Autodesk Inventor part; units mm, degrees
ref_plane "YZ Plane" through (0, 0, 0) normal (1, 0, 0) x (0, 1, 0)
ref_plane "XZ Plane" through (0, 0, 0) normal (0, 1, 0) x (-1, 0, 0)
ref_plane "XY Plane" through (0, 0, 0) normal (0, 0, 1) x (1, 0, 0)
sketch "Sketch1" plane through (0, 0, 0) normal (0, 1, 0) x (-1, 0, 0)
  line L0 (141, -70.5) -> (-141, -70.5)
  line L1 (-141, -70.5) -> (-141, 70.5)
  line L2 (-141, 70.5) -> (141, 70.5)
  line L3 (141, 70.5) -> (141, -70.5)
  line L4 (141, -70.5) -> (-141, 70.5) construction
  line L5 (-141, -70.5) -> (141, 70.5) construction
  point P0 (0, 0)
  dimension "d0" = 282
  dimension "d1" = 141
extrude "RectangleFace" add sketch "Sketch1" along normal blind 15
sketch "Sketch2" plane through (0, 15, 0) normal (0, 1, 0) x (1, 0, 0)
  line L0 (141, 70.5) -> (-141, 70.5)
  line L1 (0, 70.5) -> (0, -11.1)
  line L2 (0, -11.1) -> (-82, -11.1)
  line L3 (-122, 11.4) -> (-42, 11.4)
  line L4 (-42, 11.4) -> (-42, -33.6)
  line L5 (-42, -33.6) -> (-122, -33.6)
  line L6 (-122, -33.6) -> (-122, 11.4)
  line L7 (-122, 11.4) -> (-42, -33.6) construction
  line L8 (-42, 11.4) -> (-122, -33.6) construction
  point P0 (0, 0)
  dimension "d4" = 81.6
  dimension "d5" = 82
  dimension "d6" = 80
  dimension "d7" = 45
extrude "RectangularCut" cut sketch "Sketch2" against normal blind 15
sketch "Sketch3" plane through (0, 15, 0) normal (0, 1, 0) x (1, 0, 0)
  line L0 (-42, 11.4) -> (-122, 11.4)
  line L1 (-82, 11.4) -> (-82, 29.4)
  line L2 (-122, -33.6) -> (-42, -33.6)
  line L3 (-82, -33.6) -> (-82, -46.1)
  line L4 (-82, 29.4) -> (-74, 29.4)
  line L5 (-82, 29.4) -> (-90, 29.4)
  line L6 (-82, -46.1) -> (-74, -46.1)
  line L7 (-82, -46.1) -> (-90, -46.1)
  circle A0 centre (-74, -46.1) radius 1.75
  circle A1 centre (-90, -46.1) radius 1.75
  circle A2 centre (-74, 29.4) radius 1.75
  circle A3 centre (-90, 29.4) radius 1.75
  point P0 (0, 0)
  dimension "d10" = 18
  dimension "d11" = 12.5
  dimension "d12" = 8
  dimension "d13" = 8
  dimension "d14" = 8
  dimension "d15" = 8
  dimension "d16" = 3.5
  dimension "d17" = 3.5
  dimension "d18" = 3.5
  dimension "d19" = 3.5
extrude "AxleSupportHoles" cut sketch "Sketch3" against normal blind 15
sketch "Sketch4" plane through (0, 15, 0) normal (0, 1, 0) x (1, 0, 0)
  line L0 (141, 70.5) -> (-141, 70.5)
  line L1 (0, 70.5) -> (0, -19.5)
  line L2 (0, -19.5) -> (10, -19.5)
  line L3 (-15.5, 18.25) -> (35.5, 18.25)
  line L4 (35.5, 18.25) -> (35.5, -57.25)
  line L5 (35.5, -57.25) -> (-15.5, -57.25)
  line L6 (-15.5, -57.25) -> (-15.5, 18.25)
  line L7 (-15.5, 18.25) -> (35.5, -57.25) construction
  line L8 (35.5, 18.25) -> (-15.5, -57.25) construction
  line L9 (-15.5, 18.25) -> (-11.5, 18.25)
  line L10 (-11.5, 18.25) -> (-11.5, 14.25)
  line L11 (35.5, 18.25) -> (31.5, 18.25)
  line L12 (31.5, 18.25) -> (31.5, 14.25)
  line L13 (-15.5, -57.25) -> (-11.5, -57.25)
  line L14 (-11.5, -57.25) -> (-11.5, -53.25)
  line L15 (35.5, -57.25) -> (31.5, -57.25)
  line L16 (31.5, -57.25) -> (31.5, -53.25)
  circle A0 centre (-11.5, -53.25) radius 1.75
  circle A1 centre (31.5, -53.25) radius 1.75
  circle A2 centre (31.5, 14.25) radius 1.75
  circle A3 centre (-11.5, 14.25) radius 1.75
  point P0 (0, 0)
  dimension "d22" = 90
  dimension "d23" = 10
  dimension "d24" = 51
  dimension "d25" = 75.5
  dimension "d26" = 4
  dimension "d27" = 4
  dimension "d28" = 4
  dimension "d29" = 4
  dimension "d30" = 4
  dimension "d31" = 4
  dimension "d32" = 4
  dimension "d33" = 4
  dimension "d34" = 3.5
  dimension "d35" = 3.5
  dimension "d36" = 3.5
  dimension "d37" = 3.5
extrude "DriverHoles" cut sketch "Sketch4" against normal blind 15 contours A0 | A1 | A2 | A3
sketch "Sketch5" plane through (0, 15, 0) normal (0, 1, 0) x (1, 0, 0)
  line L0 (141, 70.5) -> (71, 70.5)
  line L1 (141, 70.5) -> (-141, 70.5)
  line L2 (71, 70.5) -> (71, 20.5)
  line L3 (71, 20.5) -> (71, -29.5)
  circle A0 centre (71, 20.5) radius 2
  circle A1 centre (71, -29.5) radius 2
  point P0 (0, 0)
  dimension "d40" = 70
  dimension "d41" = 50
  dimension "d42" = 50
  dimension "d43" = 4
  dimension "d44" = 4
extrude "Extrusion5" cut sketch "Sketch5" against normal blind 15
properties part number "RectangleFifteen1"
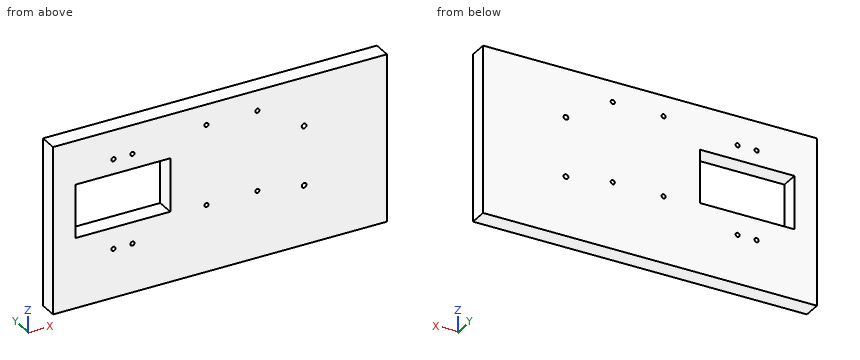
Model file for the job. Use its own axes, mm. Give positions to 0.01 mm unless a question says otherwise; leave off trailing zeros. Order: outer loops, then holes, each group sorted by start corner. A loop starts at its lowest first (then second) coordinate and runs counter-clockwise, first axis right, second up. Notation, with made-up numbers: M 63,20 L 81,20 A5 ccw 81,29 Z; hole C -6.5,28.5 d2. An arc over 180 degrees is marked long. Write item = value, one per line.
Q1. Cut at A-A, the plane y = 2.75. Count the separate pieces of the cut face and the enclosed holes in it, then the cut area to 3 significant figures.
Derived:
separate_pieces = 1
enclosed_holes = 11
area = 36,100 mm2
Q2. Cut at B-B, the plane z = 14. List the corners of the cut face in (x, y), then the cut area to 3 significant figures.
Derived:
outline = M -141,0 L -122,0 L -122,15 L -141,15 Z; M -42,0 L 141,0 L 141,15 L -42,15 Z
area = 3,030 mm2
Q3. Drill centre lines: line 1 (X direction, y = 11.75, z = 29.5); line 2 (Z direction, x = -90, y = 4); line 3 (X direction, y = 4.25, z = 53.25). Where is each one in solid material? Low to high. Write a range as [from, to].
Derived:
line_1 = [-141, -122], [-42, 69], [73, 141]
line_2 = [-70.5, -31.15], [-27.65, -11.4], [33.6, 44.35], [47.85, 70.5]
line_3 = [-141, -13.25], [-9.75, 29.75], [33.25, 141]
Q4. Cut at C-C, the plane x = -83.5. List the corners of the cut face in (y, z), then the cut area to 3 significant figures.
Derived:
outline = M 0,-70.5 L 15,-70.5 L 15,-11.4 L 0,-11.4 Z; M 0,33.6 L 15,33.6 L 15,70.5 L 0,70.5 Z
area = 1,440 mm2
Q5. Flat gauge pins, fed straight in: pin 1 (5.5 mm diameter, centred on x = -11.5, z = 53.25, fed in from +Y); pin 2 (10 mm diameter, centred on x = -50, z = 21.5, fed in from +Y). Where does each tip first touch, or does it go through?
Derived:
pin_1 = 15
pin_2 = through
